Work out the finished part from the listing and answer in its coordinate system (mm). A direction names the side the tool comes from. Round coordinates to 2 decimals unless told otherwise and drop trailing zeros. Write each loop counter-clockwise with the first axis right and the second up, starting at its lowest first coordinate (ties: lowest second). Pieces come first, ordered by that corner, then holes. Notation, with made-up numbers: (84, -25.75) -> (125, -25.75) arc R24 cw to (125, -12.75) -> close; hole circle Ø6 at (48.25, -31). An arc over 180 degrees is marked (long way). One line per item, written item: value.
```python
from build123d import *

# Parameters (mm, degrees)
F0_W     = 203.2
F0_H     = 127
F1_DEPTH = 127
F3_DEPTH = 76.2
F4_SIZE2 = 101.6
F4_SIZE  = 76.2
F5_R     = 5.08
F6_R     = 15.24
F7_DEPTH = 50.8
F8_R     = 19.252046471
F9_DEPTH = 127


with BuildPart() as f1:
    # F0 (on Front) → F1 (new body)
    with BuildSketch(Plane.XZ):
        with Locations((-4.3338742107, -2.5460490198)):
            Rectangle(F0_W, F0_H)
    extrude(amount=F1_DEPTH)

    # F2 (on face) → F3 (cut)
    with BuildSketch(Plane.XZ.offset(127)):
        Polygon((-42.4338742107, -2.5460490198), (-42.4338742107, -66.0460490198), (97.2661257893, -66.0460490198), (97.2661257893, 60.9539509802), (-4.3338742107, 60.9539509802), (-4.3338742107, -2.5460490198), align=None)
    extrude(amount=-F3_DEPTH, mode=Mode.SUBTRACT)

    # F4
    f4_edges = [f1.edges().sort_by_distance(p)[0] for p in [
        (97.266126, -25.4, 60.953951),
    ]]
    f4_side = f1.faces().sort_by_distance((-26.105303, -52.614286, 60.953951))[0]
    chamfer(f4_edges, length=F4_SIZE, length2=F4_SIZE2, reference=f4_side)

    # F5
    f5_edges = [f1.edges().sort_by_distance(p)[0] for p in [
        (-4.333874, -88.9, -2.546049),
        (-42.433874, -88.9, -2.546049),
        (-23.383874, -127, -2.546049),
        (-23.383874, -50.8, -2.546049),
        (-42.433874, 0, 60.953951),
        (21.066126, -25.4, 60.953951),
        (-105.933874, -63.5, 60.953951),
        (8.366126, -50.8, 60.953951),
        (-55.133874, -127, 60.953951),
        (-4.333874, -88.9, 60.953951),
        (-4.333874, -127, 29.203951),
        (-4.333874, -50.8, 29.203951),
        (-42.433874, -88.9, -66.046049),
        (-42.433874, -127, -34.296049),
        (-42.433874, -50.8, -34.296049),
        (97.266126, 0, -53.346049),
        (97.266126, -25.4, -40.646049),
        (97.266126, -25.4, -66.046049),
        (97.266126, -50.8, -53.346049),
        (-105.933874, -63.5, -66.046049),
        (-105.933874, 0, -2.546049),
        (-105.933874, -127, -2.546049),
        (-4.333874, 0, -66.046049),
        (27.416126, -50.8, -66.046049),
        (-74.183874, -127, -66.046049),
    ]]
    fillet(f5_edges, radius=F5_R)

    # F6 (on face) → F7 (cut, through all)
    with BuildSketch(Plane.XZ.offset(50.8)):
        with Locations((13.4461257893, -20.3260490198)):
            Circle(F6_R)
    extrude(amount=-F7_DEPTH, mode=Mode.SUBTRACT)

    # F8 (on face) → F9 (cut, through all)
    with BuildSketch(Plane.XY.offset(60.9539509802)):
        with Locations((-75.6851807237, -50.9467981756)):
            Circle(F8_R)
    extrude(amount=-F9_DEPTH, mode=Mode.SUBTRACT)


solid = f1.part
```
(1) Find section C-C on z = 14.5. Give the vertices of the cut face in (x, y).
Reported:
outline: (-105.93, -121.92) arc R5.08 ccw to (-100.85, -127) -> (-9.41, -127) arc R5.08 ccw to (-4.33, -121.92) -> (-4.33, -55.88) arc R5.08 cw to (0.75, -50.8) -> (55.91, -50.8) -> (55.91, 0) -> (-100.85, 0) arc R5.08 ccw to (-105.93, -5.08) -> close; hole circle Ø38.5 at (-75.69, -50.95)
(2) Find section D-D on y = -98. Give the vertices of the cut face in (x, z), plus the area to 3 significant figures.
Reported:
outline: (-105.93, -60.97) arc R5.08 ccw to (-100.85, -66.05) -> (-47.51, -66.05) arc R5.08 ccw to (-42.43, -60.97) -> (-42.43, -7.63) arc R5.08 cw to (-37.35, -2.55) -> (-9.41, -2.55) arc R5.08 ccw to (-4.33, 2.53) -> (-4.33, 55.87) arc R5.08 ccw to (-9.41, 60.95) -> (-100.85, 60.95) arc R5.08 ccw to (-105.93, 55.87) -> close
area: 10,500 mm2
(3) A tool of negligible diameter and unlimited length cuts with its end or side. For faces 1 (the face through (9.96, -49.27, 59.51)), 2 (the face through (-40.985, -88.438, -4.074)), 3 (the face through (-4.334, -89, 30)), 4 (the face through (-54.49, -125.47, 59.51)), from which of +Z, -Z, +X, -X, +Y, -Y can it reach the whole face along a straight path? Write none if from no direction.
Reported:
face 1: +Z, +X, -Y
face 2: -Z, +X, -Y
face 3: +Z, -Z, +X, -Y
face 4: +Z, +X, -X, -Y
(4) Find section B-B on x = -14. Give the vertices of the cut face in (y, z), plus the area to 3 significant figures.
Reported:
outline: (-127, 2.53) arc R5.08 ccw to (-121.92, -2.55) -> (-55.88, -2.55) arc R5.08 cw to (-50.8, -7.63) -> (-50.8, -60.97) arc R5.08 ccw to (-45.72, -66.05) -> (-5.08, -66.05) arc R5.08 ccw to (0, -60.97) -> (0, 55.87) arc R5.08 ccw to (-5.08, 60.95) -> (-121.92, 60.95) arc R5.08 ccw to (-127, 55.87) -> close
area: 11,300 mm2
(5) Consider probe 1 along Z at (x, y) = (13, -22); probe 2 along Y at (x, z) = (72.5, -43.5); probe 3 along X at (y, z) = (-82.5, 7). Determine where each line is inside the solid, lowest interval first.
Reported:
probe 1: z = -66.05 to -35.56, -5.09 to 60.95
probe 2: y = -50.8 to 0
probe 3: x = -105.93 to -4.33
(6) Find section A-A on y = -43. Give the vertices of the cut face in (x, z).
Reported:
outline: (-105.93, -60.97) arc R5.08 ccw to (-100.85, -66.05) -> (-93.22, -66.05) -> (-93.22, 60.95) -> (-100.85, 60.95) arc R5.08 ccw to (-105.93, 55.87) -> close; (-58.15, -66.05) -> (92.19, -66.05) arc R5.08 ccw to (97.27, -60.97) -> (97.27, -42.34) arc R5.08 ccw to (96.25, -39.29) -> (22.59, 58.92) arc R5.08 ccw to (18.53, 60.95) -> (-58.15, 60.95) -> close; hole circle Ø30.48 at (13.45, -20.33)
(7) Flat-ended cylindrical pins translate along their axes: pin 1 Ø16 at (y, z) = (-77.5, -36) entering from +X; pin 2 Ø16 at (y, z) = (-87.5, 36) entering from +X; pin 3 Ø14 at (x, y) = (-28, -83.5) entering from -Z. Find the tip coordinate at first contact, or state that the pin passes through.
Reported:
pin 1: stops at x = -42.43
pin 2: stops at x = -4.33
pin 3: stops at z = -2.55
